from build123d import *

# Parameters (mm, degrees)
F1_DEPTH = 5.842
F0_W     = 36.9333177805
F0_H     = 90.6793028116
F2_DEPTH = 5.588


with BuildPart() as f1:
    # F0 (on Front) → F1 (new body)
    with BuildSketch(Plane.XZ):
        with BuildLine():
            Line((-54.8489093781, 90.6793028116), (-17.9155915976, 90.6793028116))
            ThreePointArc((-17.9155915976, 90.6793028116), (-36.3822504878, 220.1306557061), (-54.8489093781, 90.6793028116))
        make_face()
    extrude(amount=F1_DEPTH)

    # F0 (on Front) → F2 (join)
    with BuildSketch(Plane.XZ):
        with Locations((-36.3822504878, 45.3396514058)):
            Rectangle(F0_W, F0_H)
    extrude(amount=F2_DEPTH)


solid = f1.part
Geometry: final body of the model. Coordinates: model frame, mm. A direction names the side the tool comes from. Round coordinates to 2 decimals unless told otherwise and drop trailing zeros. Order: outer loops, then holes, each group sorted by start corner. A loop starts at its lowest first (then second) coordinate and runs counter-clockwise, first axis right, second up. Notation, with made-up numbers: (-32.75, 32) -> (10.25, 32) arc R26 ccw to (10.25, 47) -> close; hole circle Ø8 at (-30, 85.25). An arc over 180 degrees is marked (long way). Put each result on its own line as item: value. Start each with the question number.
Q1. Section B-B on z = 48.5. Return the cut outline in (x, y).
Q2. First-contact query: pin 1 (1 mm diameter, centred on y = -2, z = 43, fed in from +X); pin 2 (8 mm diameter, centred on x = -52, z = 39, fed in from -Y); pin 3 (2 mm diameter, centred on x = 1.5, y = -3.5, fed in from +Z). Flat tips, straight axial feed; report the tip coordinate or a pass-through.
Q3. Reachability of faces 1 (the flat face through (-17.916, -3, 45)), 2 (the flat face through (-54.849, -3, 45)), 3 (the flat face through (-37, -5.588, 46)) from +Z, -Z, +X, -X, +Y, -Y: full face, straight path, thin tool, end or side. Return the list, or none.
Q4. Section A-A on y = -1.9. Return the cut outline in (x, z), and give its area (3 significant figures).
Q5. Line query: probe 1 along X at (y, z) = (-4, 19); probe 2 along X at (y, z) = (-1.2, 153); probe 3 along Y at (x, z) = (-49.5, 37.5). Output: solid intervals per line, ascending.
Ans:
1. outline: (-54.85, -5.59) -> (-17.92, -5.59) -> (-17.92, 0) -> (-54.85, 0) -> close
2. pin 1: stops at x = -17.92
2. pin 2: stops at y = -5.59
2. pin 3: stops at z = 208.87
3. face 1: -Z, +X, +Y, -Y
3. face 2: -Z, -X, +Y, -Y
3. face 3: -Z, +X, -X, -Y
4. outline: (-54.85, 0) -> (-17.92, 0) -> (-17.92, 90.68) arc R66.04 ccw (long way) to (-54.85, 90.68) -> close
4. area: 17,000 mm2
5. probe 1: x = -54.85 to -17.92
5. probe 2: x = -102.42 to 29.65
5. probe 3: y = -5.59 to 0
